Build history of the part. All positions in model axes, mm. A direction names the side the tool comes from. Round coordinates to 2 decimals unless told otherwise and drop trailing zeros. Write each loop counter-clockwise with the first axis right and the second up, starting at its lowest first coordinate (ties: lowest second). Pieces come first, ordered by that corner, then holes.
Autodesk Inventor part; units mm, degrees
ref_plane "YZ Plane" through (0, 0, 0) normal (1, 0, 0) x (0, 1, 0)
ref_plane "XZ Plane" through (0, 0, 0) normal (0, 1, 0) x (-1, 0, 0)
ref_plane "XY Plane" through (0, 0, 0) normal (0, 0, 1) x (1, 0, 0)
sketch "Boceto1" plane through (0, 0, 0) normal (0, 0, 1) x (1, 0, 0)
  circle A0 centre (0, 0) radius 20
  circle A1 centre (0, 0) radius 12.7 construction
  line L0 (0, 12.7) -> (8.9803, 8.9803)
  line L1 (8.9803, 8.9803) -> (12.7, 0)
  line L2 (12.7, 0) -> (8.9803, -8.9803)
  line L3 (8.9803, -8.9803) -> (0, -12.7)
  line L4 (0, -12.7) -> (-8.9803, -8.9803)
  line L5 (-8.9803, -8.9803) -> (-12.7, 0)
  line L6 (-12.7, 0) -> (-8.9803, 8.9803)
  line L7 (-8.9803, 8.9803) -> (0, 12.7)
  dimension "d1" = 25.4
  dimension "d0" = 40
extrude "Extrusión1" add sketch "Boceto1" along normal blind 1.5
properties part number "espaciador1.5mm"
1) Slice it at B-B (z = 0.3). Write the cut outline in (x, y).
Results:
outline: circle Ø40 at (0, 0); hole (-12.7, 0) - (-8.98, -8.98) - (0, -12.7) - (8.98, -8.98) - (12.7, 0) - (8.98, 8.98) - (0, 12.7) - (-8.98, 8.98) - close
2) Slice it at C-C (y = 8). Write the cut outline in (x, z), plus the area to 3 significant figures.
Results:
outline: (-18.33, 0) - (-9.39, 0) - (-9.39, 1.5) - (-18.33, 1.5) - close; (9.39, 0) - (18.33, 0) - (18.33, 1.5) - (9.39, 1.5) - close
area: 26.8 mm2
3) Pin check, flat tip, straight feed: pin 1 Ø10 at (x, y) = (-2.5, 0) entering from +Z. Stop position of the tip, or through.
Results:
pin 1: passes through
4) Mould opens along X. For faces 1 (the flat face through (4.553, -10.814, 0.74)), 2 (the flat face through (13, 0, 1.5)), 3 (the cylindrical face through (-4.336, 19.524, 0.74)) say: released by +X, released by -X, zero draft, split by the parting line, or undercut.
Results:
face 1: undercut
face 2: zero draft
face 3: split by the parting line
5) Wall check: L1, parallel to Y at x = 4, z = 0.85; L2, parallel to Y at x = -11, z = 0.9. Give the ranges that are in metal, low to high.
Results:
L1: y = -19.6 to -11.04, 11.04 to 19.6
L2: y = -16.7 to -4.1, 4.1 to 16.7
6) Slice it at D-D (x = -13.5). Write the cut outline in (y, z).
Results:
outline: (-14.76, 0) - (14.76, 0) - (14.76, 1.5) - (-14.76, 1.5) - close
7) Slice it at A-A (x = 11). Write the cut outline in (y, z).
Results:
outline: (-16.7, 0) - (-4.1, 0) - (-4.1, 1.5) - (-16.7, 1.5) - close; (4.1, 0) - (16.7, 0) - (16.7, 1.5) - (4.1, 1.5) - close
8) Which spindle directions (+Z, -Z, +X, -X, +Y, -Y) get a long thin tool onto all of the face, cutting with end or side? Do faces 4 (the flat face through (-10.866, 4.427, 0.74)), 5 (the flat face through (13, 0, 0)). Say none if no direction does.
Results:
face 4: +Z, -Z
face 5: -Z, +X, -X, +Y, -Y
